CAD build for the part. Positions are in the model's coordinates, mm. Round coordinates to 2 decimals unless told otherwise and drop trailing zeros. Loops run counter-clockwise (first coordinate to the right, second up) from the corner with the lowest first, then second, coordinate; pieces in that order, holes last.
```python
from build123d import *

# Parameters (mm, degrees)
F0_W     = 72.1
F0_H     = 142.4
F1_DEPTH = 8.3
F2_R     = 5.08
F3_R     = 5.08


with BuildPart() as f1:
    # F0 (on Front) → F1 (new body)
    with BuildSketch(Plane.XZ):
        Rectangle(F0_W, F0_H)
    extrude(amount=F1_DEPTH)

    # F2
    f2_edges = [f1.edges().sort_by_distance(p)[0] for p in [
        (-36.05, -4.15, 71.2),
        (36.05, -4.15, 71.2),
        (36.05, -4.15, -71.2),
        (-36.05, -4.15, -71.2),
    ]]
    fillet(f2_edges, radius=F2_R)

    # F3
    f3_edges = [f1.edges().sort_by_distance(p)[0] for p in [
        (36.05, 0, 0),
    ]]
    fillet(f3_edges, radius=F3_R)


solid = f1.part
```
Item 1: Cut at B-B, the plane y = -2.75. Give the cut face in (x, z).
Answers follow:
outline: (-35.48, -66.12) arc R4.51 ccw to (-30.97, -70.63) - (30.97, -70.63) arc R4.51 ccw to (35.48, -66.12) - (35.48, 66.12) arc R4.51 ccw to (30.97, 70.63) - (-30.97, 70.63) arc R4.51 ccw to (-35.48, 66.12) - close
Item 2: Probe line 1 (X direction, y = -4.75, z = 5); line 2 (Z direction, x = 25, y = -4); line 3 (X direction, y = -1.5, z = -61). List the from-to ranges inside material, lowest first.
Answers follow:
line 1: x = -36.04 to 36.04
line 2: z = -71.08 to 71.08
line 3: x = -34.57 to 34.57
Item 3: Cut at A-A, the plane z = -18. Give the cut face in (x, y), plus the area to 3 significant figures.
Answers follow:
outline: (-36.05, -8.3) - (36.05, -8.3) - (36.05, -5.08) arc R5.08 ccw to (30.97, 0) - (-30.97, 0) arc R5.08 ccw to (-36.05, -5.08) - close
area: 587 mm2
Item 4: Flat gauge pin, fed straight in: P1, Ø3, axis at y = -3, z = -11, coming from the +X side. Where does the tip first touch, or does it go through?
Answers follow:
P1: stops at x = 36.02
